Could you check a few things on this model? Use its own coordinates, in mm. Face numbers are marked on the shaded views. A direction names the side the tool comes from. Give positions to 0.01 mm unless a question says otherwise; leave off trailing zeros. Order: outer loops, then holes, each group sorted by start corner. A loop starts at its lowest first (then second) coordinate and runs counter-clockwise, first axis right, second up. Notation, with made-up numbers: M 11.25,24.25 L 27.25,24.25 A17 cw 27.25,38.25 Z; hole C 78.5,5 d9. An arc over 180 degrees is marked long. Answer in a Markdown table with one row per item. Add a question column.
```python
from build123d import *

# Parameters (mm, degrees)
SKETCH004_W  = 140.699818
SKETCH004_H  = 7
PAD007_DEPTH = 17
SKETCH006_W  = 100
SKETCH006_H  = 10
PAD005_DEPTH = 20
SKETCH005_R  = 22
PAD006_DEPTH = 17
SKETCH007_R  = 25.5
PAD004_DEPTH = 20
FILLET014_R  = 2
FILLET015_R  = 2
FILLET016_R  = 2
FILLET017_R  = 2
FILLET018_R  = 2
FILLET019_R  = 2


with BuildPart() as body007:
    # Sketch004 → Pad007 (new body)
    with BuildSketch(Plane.XY):
        with Locations((8.122221, 0)):
            Rectangle(SKETCH004_W, SKETCH004_H)
    extrude(amount=PAD007_DEPTH)


with BuildPart() as body007_1:
    # Body007 placement: moved
    add(body007.part.moved(Location((0, 0, 3))))


with BuildPart() as body004:
    # Sketch006 → Pad005 (new body)
    with BuildSketch(Plane.XY):
        Rectangle(SKETCH006_W, SKETCH006_H)
    extrude(amount=PAD005_DEPTH)


with BuildPart() as cut001:
    # Sketch005 → Pad006 (new body)
    with BuildSketch(Plane.XY):
        Circle(SKETCH005_R)
    extrude(amount=PAD006_DEPTH)

    # Cut001: cut Body004
    add(body004.part, mode=Mode.SUBTRACT)


with BuildPart() as fillet019:
    # Sketch007 → Pad004 (new body)
    with BuildSketch(Plane.XY):
        Circle(SKETCH007_R)
    extrude(amount=PAD004_DEPTH)

    # Cut002: cut Cut001
    add(cut001.part, mode=Mode.SUBTRACT)

    # Cut003: cut Body007
    add(body007_1.part, mode=Mode.SUBTRACT)


with BuildPart() as fillet019_1:
    # Cut003 placement: moved
    add(fillet019.part.moved(Location((25.5, 0, 0))))

    # Fillet014
    fillet014_edges = [fillet019_1.edges().sort_by_distance(p)[0] for p in [
        (25.5, -25.5, 20),
    ]]
    fillet(fillet014_edges, radius=FILLET014_R)

    # Fillet015
    fillet015_edges = [fillet019_1.edges().sort_by_distance(p)[0] for p in [
        (25.5, 25.5, 20),
    ]]
    fillet(fillet015_edges, radius=FILLET015_R)

    # Fillet016
    fillet016_edges = [fillet019_1.edges().sort_by_distance(p)[0] for p in [
        (25.5, -22, 17),
    ]]
    fillet(fillet016_edges, radius=FILLET016_R)

    # Fillet017
    fillet017_edges = [fillet019_1.edges().sort_by_distance(p)[0] for p in [
        (25.5, 22, 17),
    ]]
    fillet(fillet017_edges, radius=FILLET017_R)

    # Fillet018
    fillet018_edges = [fillet019_1.edges().sort_by_distance(p)[0] for p in [
        (25.5, -5, 17),
    ]]
    fillet(fillet018_edges, radius=FILLET018_R)

    # Fillet019
    fillet019_edges = [fillet019_1.edges().sort_by_distance(p)[0] for p in [
        (25.5, 5, 17),
    ]]
    fillet(fillet019_edges, radius=FILLET019_R)


solid = fillet019_1.part
```
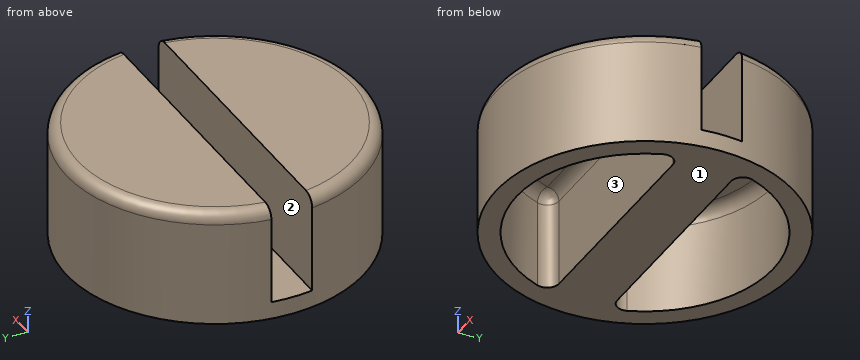
1. Suppose I cut it at A-A on z = 9. List the corners of the cut face in (x, y) for me (1 decimal).
2. Suppose I cut it at D-D on z = 16. Count the separate pieces of the cut face and the enclosed holes in it, plus the area to 3 significant figures.
3. Suppose I cut it at C-C on y = 0. List the corners of the cut face in (x, z) for me.
4. For the marked faces 1, 2 and 3, which set-ups out of +Z, -Z, +X, -X, +Y, -Y let a thin tool reach every point of the face, with its end or its side?
5. Will these pins go through, and if not, where does the flat tip stop? P1, Ø1, axis at x = 5.5, z = 3, coming from the +Y side; P2, Ø6, axis at y = -1.5, z = 15.5, coming from the +X side; P3, Ø7.5, axis at x = 21.5, z = 5, coming from the -Y side.
6. If I drill on line 1 along Y through (x, z) = (27, 8.75); line 2 along Y through (x, z) = (29, 11.75); line 3 along Y through (x, z) = (23.5, 2.5), over which ranges is the centre line in solid material (lowest first)? Write a range as [from, to].
7. Suppose I cut it at B-B on x = 25.5. List the corners of the cut face in (y, z) for me, plus the area to 3 significant figures.
Findings below:
| question | item | result |
|---|---|---|
| 1 | outline | M 0.2,-3.5 A25.5 ccw 50.8,-3.5 Z; M 0.2,3.5 L 50.8,3.5 A25.5 ccw Z; hole M 4.9,-7.7 A22 ccw 46.1,-7.7 A2 ccw 44.2,-5 L 6.8,-5 A2 ccw Z; hole M 4.9,7.7 A2 ccw 6.8,5 L 44.2,5 A2 ccw 46.1,7.7 A22 ccw Z |
| 2 | separate pieces | 2 |
| 2 | enclosed holes | 2 |
| 2 | area | 662 mm2 |
| 3 | outline | M 0,0 L 51,0 L 51,3 L 0,3 Z |
| 4 | face 1 | -Z, +X, -X, +Y, -Y |
| 4 | face 2 | +Z, +X, -X |
| 4 | face 3 | -Z |
| 5 | P1 | y = 16.43 |
| 5 | P2 | x = 50.76 |
| 5 | P3 | y = -25.5 |
| 6 | line 1 | [-25.46, -21.95], [-5, -3.5], [3.5, 5], [21.95, 25.46] |
| 6 | line 2 | [-25.26, -21.72], [-5, -3.5], [3.5, 5], [21.72, 25.26] |
| 6 | line 3 | [-25.42, -21.91], [-5, 5], [21.91, 25.42] |
| 7 | outline | M -25.5,0 L -22,0 L -22,15 A2 cw -20,17 L -7,17 A2 cw -5,15 L -5,0 L 5,0 L 5,15 A2 cw 7,17 L 20,17 A2 cw 22,15 L 22,0 L 25.5,0 L 25.5,18 A2 ccw 23.5,20 L 3.5,20 L 3.5,3 L -3.5,3 L -3.5,20 L -23.5,20 A2 ccw -25.5,18 Z |
| 7 | area | 325 mm2 |
